Can you work these out from the model? Positions are in its coordinate system, mm. Face numbers are marked on the shaded views. A direction names the side the tool comes from. Coordinates: 2 decimals unless noted, no trailing zeros. Loops run counter-clockwise (first coordinate to the right, second up) from the corner with the lowest first, then second, coordinate; pieces in that order, holes last. Notation, with made-up numbers: (37, 56) - (55, 56) arc R19 cw to (55, 91) - close; hole circle Ø1 at (4, 51). An arc over 180 degrees is marked (long way). Put each result on its own line as item: value. Start each with the question number.
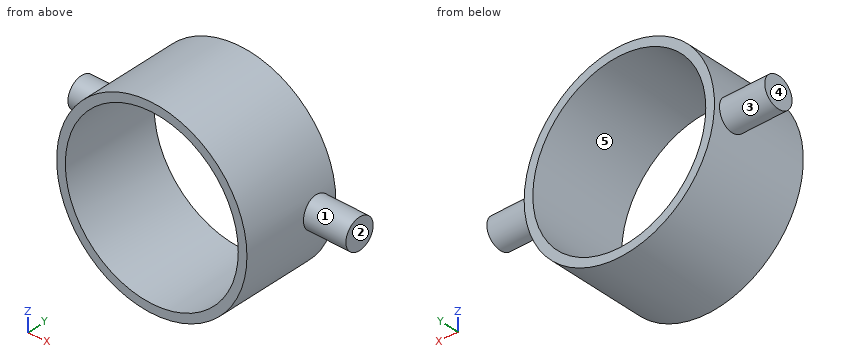
from build123d import *

# Parameters (mm, degrees)
F0_R     = 3.4257116129
F0_R_2   = 3.1136968268
F1_DEPTH = 3.556
F3_START = 3.2004
F2_R     = 0.5461
F3_DEPTH = 1.7526
F4_START = -3.175
F4_DEPTH = 1.8796


with BuildPart() as f1:
    # F0 (on Front) → F1 (new body)
    with BuildSketch(Plane.XZ):
        Circle(F0_R)
        Circle(F0_R_2, mode=Mode.SUBTRACT)
    extrude(amount=F1_DEPTH)

    # F2 (on Right) → F3 (join)
    with BuildSketch(Plane.YZ.offset(F3_START)):
        with Locations((-0.7492110241, 0)):
            Circle(F2_R)
    extrude(amount=F3_DEPTH)

    # F2 (on Right) → F4 (join)
    with BuildSketch(Plane.YZ.offset(F4_START)):
        with Locations((-0.7492110241, 0)):
            Circle(F2_R)
    extrude(amount=-F4_DEPTH)


solid = f1.part
Q1. I want a section at B-B on x = 0. List the corners of the cut face in (y, z) for me, and give its area (3 significant figures).
Q2. On a 3-axis mill with a long thin cutter (end or side, diameter ignored), from which of +Z, -Z, +X, -X, +Y, -Y can I reach the whole of each face in a straight line? I mean the marked faces 1 and 2. Say none if no direction works.
Q3. Please list where these lines run through material, in increasing order: line 1 along Z through (x, y) = (0, -2.7); line 2 along X through (y, z) = (-0.5, -1.5). Write a range as [from, to].
Q4. We'd pull the mould along Z, two halves only. Please class the marked faces 3, 4 and 5: released by +Z, released by -Z, zero draft, split by the parting line, or undercut.
Q5. I want a section at C-C on z = -3. List the corners of the cut face in (x, y) for me.
Q6. Will these pins go through, and if not, where does the flat tip stop? pin 1 (2 mm diameter, centred on y = -1.5, z = 1.5, fed in from -X); pin 2 (2 mm diameter, centred on y = -2, z = -0.5, fed in from +X).
Q7. I want a section at D-D on x = -3.75. List the corners of the cut face in (y, z) for me.
Q8. I want a section at A-A on z = 0. List the corners of the cut face in (x, y) for me.
Calculated:
1. outline: (-3.56, -3.43) - (0, -3.43) - (0, -3.11) - (-3.56, -3.11) - close; (-3.56, 3.11) - (0, 3.11) - (0, 3.43) - (-3.56, 3.43) - close
1. area: 2.22 mm2
2. face 1: +X
2. face 2: +Z, -Z, +X, +Y, -Y
3. line 1: [-3.43, -3.11], [3.11, 3.43]
3. line 2: [-3.08, -2.73], [2.73, 3.08]
4. face 3: split by the parting line
4. face 4: zero draft
4. face 5: undercut
5. outline: (-1.65, -3.56) - (-0.83, -3.56) - (-0.83, 0) - (-1.65, 0) - close; (0.83, -3.56) - (1.65, -3.56) - (1.65, 0) - (0.83, 0) - close
6. pin 1: x = -3.39
6. pin 2: x = 4.95
7. outline: circle Ø1.09 at (-0.75, 0)
8. outline: (-5.05, -1.3) - (-3.43, -1.3) - (-3.43, -3.56) - (-3.11, -3.56) - (-3.11, 0) - (-3.43, 0) - (-3.43, -0.2) - (-5.05, -0.2) - close; (3.11, -3.56) - (3.43, -3.56) - (3.43, -1.3) - (4.95, -1.3) - (4.95, -0.2) - (3.43, -0.2) - (3.43, 0) - (3.11, 0) - close
